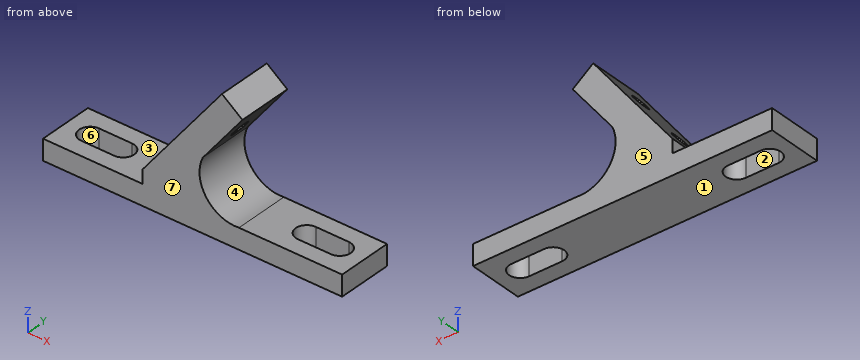
```python
from build123d import *

# Parameters (mm, degrees)
EXTRUDE_1_DEPTH     = 8
CUT_EXTRUDE_1_REACH = 22.104
SKETCH_3_R          = 1.25
CUT_EXTRUDE_2_DEPTH = 6


with BuildPart() as part:
    # Эскиз1 → Бобышка-Вытянуть1 (new body)
    with BuildSketch(Plane(origin=(0, 0, 0), x_dir=(1, 0, 0), z_dir=(0, 1, 0))):
        with BuildLine():
            Line((-21.75, 0), (21.75, 0))
            Line((21.75, 0), (21.75, -3))
            Line((21.75, -3), (6.75, -3))
            ThreePointArc((6.75, -3), (1.985016763, -5.099789535), (1.486609174, -10.283009694))
            Line((1.486609174, -10.283009694), (7.25, -17.835050888))
            Line((7.25, -17.835050888), (4.276781652, -20.104082387))
            Line((4.276781652, -20.104082387), (-7.25, -5))
            Line((-7.25, -5), (-7.25, -3))
            Line((-7.25, -3), (-21.75, -3))
            Line((-21.75, -3), (-21.75, 0))
        make_face()
    extrude(amount=EXTRUDE_1_DEPTH)

    # Эскиз2 → Вырез-Вытянуть1 (cut, up to next)
    with BuildSketch(Plane(origin=(0, 0, 0), x_dir=(-1, 0, 0), z_dir=(0, 0, -1)), mode=Mode.PRIVATE) as cut_extrude_1_sk1:
        with BuildLine():
            Line((-18.15, 5.6), (-13.35, 5.6))
            ThreePointArc((-13.35, 5.6), (-11.75, 4), (-13.35, 2.4))
            Line((-13.35, 2.4), (-18.15, 2.4))
            ThreePointArc((-18.15, 2.4), (-19.75, 4), (-18.15, 5.6))
        make_face()
    cut_extrude_1_tool1 = extrude(cut_extrude_1_sk1.sketch, amount=-CUT_EXTRUDE_1_REACH, mode=Mode.PRIVATE) & part.part
    add(cut_extrude_1_tool1.solids().sort_by_distance((15.75, 4, 0))[0], mode=Mode.SUBTRACT)
    # Эскиз2 → Вырез-Вытянуть1 (cut, up to next)
    with BuildSketch(Plane(origin=(0, 0, 0), x_dir=(-1, 0, 0), z_dir=(0, 0, -1)), mode=Mode.PRIVATE) as cut_extrude_1_sk2:
        with BuildLine():
            Line((18.15, 5.6), (13.35, 5.6))
            ThreePointArc((13.35, 5.6), (11.75, 4), (13.35, 2.4))
            Line((13.35, 2.4), (18.15, 2.4))
            ThreePointArc((18.15, 2.4), (19.75, 4), (18.15, 5.6))
        make_face()
    cut_extrude_1_tool2 = extrude(cut_extrude_1_sk2.sketch, amount=-CUT_EXTRUDE_1_REACH, mode=Mode.PRIVATE) & part.part
    add(cut_extrude_1_tool2.solids().sort_by_distance((-15.75, 4, 0))[0], mode=Mode.SUBTRACT)

    # Эскиз3 → Вырез-Вытянуть2 (cut)
    with BuildSketch(Plane(origin=(-6.9930021, 0, 5.336756397), x_dir=(0.606672719, 0, 0.794951705), z_dir=(-0.794951705, 0, 0.606672719))):
        with Locations((12.576381314, 4)):
            Circle(SKETCH_3_R)
        with Locations((3.076381314, 4)):
            Circle(SKETCH_3_R)
    extrude(amount=-CUT_EXTRUDE_2_DEPTH, mode=Mode.SUBTRACT)


solid = part.part
```
Geometry: final body of the model. Coordinates: model frame, mm. Face numbers are marked on the shaded views. A direction names the side the tool comes from. Give positions to 0.01 mm unless a question says otherwise; leave off trailing zeros. Order: outer loops, then holes, each group sorted by start corner. A loop starts at its lowest first (then second) coordinate and runs counter-clockwise, first axis right, second up. Notation, with made-up numbers: (10, 75.25) -> (54, 75.25) arc R18 ccw to (54, 86.25) -> close; hole circle Ø2 at (42.25, -4). An arc over 180 degrees is marked (long way). Write each question's results on one line, items separated by ' | '. Start each with the question number.
1) Draft query along Y for the marked faces 4, 5, 6 and 7. Return one class per face: pulls with the +Y half, pulls with the -Y half, needs draft (parallel to the pull), parting line crosses it, or undercut.
2) Line query: line 1 (X direction, y = 3.25, z = 1); line 2 (Z direction, x = 7, y = 0.75); line 3 (Z direction, x = 0, y = 3.25). Output: solid intervals per line, ascending. Write a range as from..to.
3) Section C-C (y = 4). Return loops of the section in (x, z).
4) Set-up query: the marked faces 1, 2 and 3. Return all of +Z, -Z, +X, -X, +Y, -Y with unobstructed straight access to the full face (end or side cutting, diameter ignored); none if empty.
5) Section B-B (z = 1.5). Return loops of the section in (x, y).
6) Section A-A (x = 14). Return loops of the section in (y, z), then the cut area to 3 significant figures.
7) Section D-D (x = 6). Return loops of the section in (y, z).
8) First-contact query: pin 1 (4 mm diameter, centred on x = 14, y = 6, fed in from +Z); pin 2 (1 mm diameter, centred on y = 3.5, z = 4, fed in from -X); pin 3 (1.5 mm diameter, centred on x = 0.5, y = 2.5, fed in from +Z). Flat tips, straight axial feed; report the tip coordinate or a pass-through.
Calculated:
1) face 4: needs draft | face 5: pulls with the +Y half | face 6: undercut | face 7: pulls with the -Y half
2) line 1: -21.75..-19.56, -11.94..11.94, 19.56..21.75 | line 2: 0..3, 17.51..18.03 | line 3: 0..4.61, 5.13..14.5
3) outline: (-21.75, 0) -> (-19.75, 0) -> (-19.75, 3) -> (-21.75, 3) -> close; (-11.75, 0) -> (11.75, 0) -> (11.75, 3) -> (6.75, 3) arc R5.15 cw to (1.49, 10.28) -> (2.85, 12.07) -> (-0.12, 14.34) -> (-4.37, 8.78) -> (0.4, 5.14) -> (-1.12, 3.15) -> (-5.88, 6.79) -> (-7.25, 5) -> (-7.25, 3) -> (-11.75, 3) -> close; (1.4, 16.33) -> (4.37, 14.06) -> (7.25, 17.84) -> (4.28, 20.1) -> close; (19.75, 0) -> (21.75, 0) -> (21.75, 3) -> (19.75, 3) -> close
4) face 1: -Z, +X, -X, +Y, -Y | face 2: +Z, -Z | face 3: +Z, -X, +Y, -Y
5) outline: (-21.75, 0) -> (21.75, 0) -> (21.75, 8) -> (-21.75, 8) -> close; hole (-18.15, 2.4) -> (-13.35, 2.4) arc R1.6 ccw to (-13.35, 5.6) -> (-18.15, 5.6) arc R1.6 ccw to start; hole (13.35, 2.4) -> (18.15, 2.4) arc R1.6 ccw to (18.15, 5.6) -> (13.35, 5.6) arc R1.6 ccw to start
6) outline: (0, 0) -> (2.4, 0) -> (2.4, 3) -> (0, 3) -> close; (5.6, 0) -> (8, 0) -> (8, 3) -> (5.6, 3) -> close | area: 14.4 mm2
7) outline: (0, 0) -> (8, 0) -> (8, 2.97) -> (0, 2.97) -> close; (0, 16.2) -> (8, 16.2) -> (8, 18.79) -> (0, 18.79) -> close
8) pin 1: z = 3 | pin 2: x = -7.25 | pin 3: z = 16.14
